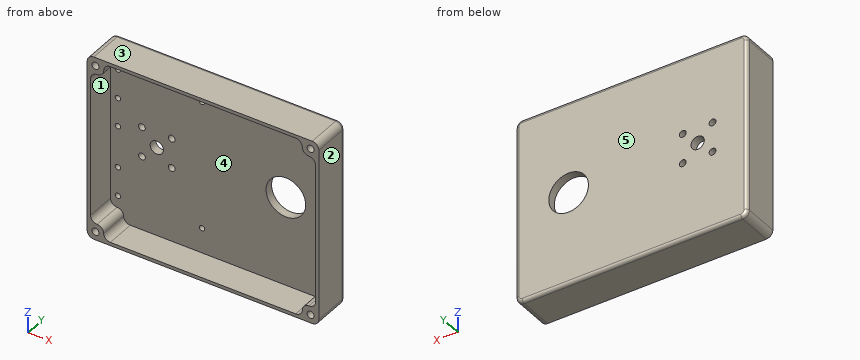
```python
from build123d import *

# Parameters (mm, degrees)
SKETCH2_R           = 3.3734375
BOSS_EXTRUDE1_DEPTH = 28.575
SKETCH2_3_R         = 19.05
SKETCH2_3_R_2       = 3.2639
SKETCH2_3_R_3       = 6.35
BOSS_EXTRUDE2_DEPTH = 7.9375
FILLET1_R           = 3.175
SKETCH3_R           = 2.57937
CUT_EXTRUDE1_DEPTH  = 4.7625


with BuildPart() as part:
    # Sketch2 → Boss-Extrude1 (new body)
    with BuildSketch(Plane(origin=(0, 0, 0), x_dir=(1, 0, 0), z_dir=(0, 1, 0))):
        with BuildLine():
            Line((104.775, -88.9), (-104.775, -88.9))
            ThreePointArc((-104.775, -88.9), (-109.265128061, -87.040128061), (-111.125, -82.55))
            Line((-111.125, -82.55), (-111.125, 82.55))
            ThreePointArc((-111.125, 82.55), (-109.265128061, 87.040128061), (-104.775, 88.9))
            Line((-104.775, 88.9), (104.775, 88.9))
            ThreePointArc((104.775, 88.9), (109.265128061, 87.040128061), (111.125, 82.55))
            Line((111.125, 82.55), (111.125, -82.55))
            ThreePointArc((111.125, -82.55), (109.265128061, -87.040128061), (104.775, -88.9))
        make_face()
        with Locations((-103.1875, -80.9625)):
            Circle(SKETCH2_R, mode=Mode.SUBTRACT)
        with Locations((-103.1875, 80.9625)):
            Circle(SKETCH2_R, mode=Mode.SUBTRACT)
        with Locations((103.1875, 80.9625)):
            Circle(SKETCH2_R, mode=Mode.SUBTRACT)
        with Locations((103.1875, -80.9625)):
            Circle(SKETCH2_R, mode=Mode.SUBTRACT)
        with BuildLine():
            Line((-107.95, -66.675), (-107.95, 66.772716465))
            ThreePointArc((-107.95, 66.772716465), (-106.090128061, 71.262844526), (-101.6, 73.122716465))
            ThreePointArc((-101.6, 73.122716465), (-97.178967915, 74.953967915), (-95.347716465, 79.375))
            ThreePointArc((-95.347716465, 79.375), (-93.487844526, 83.865128061), (-88.997716465, 85.725))
            Line((-88.997716465, 85.725), (88.9, 85.725))
            ThreePointArc((88.9, 85.725), (93.390128061, 83.865128061), (95.25, 79.375))
            ThreePointArc((95.25, 79.375), (97.109871939, 74.884871939), (101.6, 73.025))
            ThreePointArc((101.6, 73.025), (106.090128061, 71.165128061), (107.95, 66.675))
            Line((107.95, 66.675), (107.95, -66.675))
            ThreePointArc((107.95, -66.675), (106.090128061, -71.165128061), (101.6, -73.025))
            ThreePointArc((101.6, -73.025), (97.109871939, -74.884871939), (95.25, -79.375))
            ThreePointArc((95.25, -79.375), (93.390128061, -83.865128061), (88.9, -85.725))
            Line((88.9, -85.725), (-88.9, -85.725))
            ThreePointArc((-88.9, -85.725), (-93.390128061, -83.865128061), (-95.25, -79.375))
            ThreePointArc((-95.25, -79.375), (-97.109871939, -74.884871939), (-101.6, -73.025))
            ThreePointArc((-101.6, -73.025), (-106.090128061, -71.165128061), (-107.95, -66.675))
        make_face(mode=Mode.SUBTRACT)
    extrude(amount=-BOSS_EXTRUDE1_DEPTH)

    # Sketch2<3> → Boss-Extrude2 (add)
    with BuildSketch(Plane(origin=(0, 0, 0), x_dir=(1, 0, 0), z_dir=(0, 1, 0))):
        with BuildLine():
            Line((-104.775, -88.9), (104.775, -88.9))
            ThreePointArc((104.775, -88.9), (109.265128061, -87.040128061), (111.125, -82.55))
            Line((111.125, -82.55), (111.125, 82.55))
            ThreePointArc((111.125, 82.55), (109.265128061, 87.040128061), (104.775, 88.9))
            Line((104.775, 88.9), (-104.775, 88.9))
            ThreePointArc((-104.775, 88.9), (-109.265128061, 87.040128061), (-111.125, 82.55))
            Line((-111.125, 82.55), (-111.125, -82.55))
            ThreePointArc((-111.125, -82.55), (-109.265128061, -87.040128061), (-104.775, -88.9))
        make_face()
        with Locations((60.325, 0)):
            Circle(SKETCH2_3_R, mode=Mode.SUBTRACT)
        with Locations((-77.7875, -14.2875)):
            Circle(SKETCH2_3_R_2, mode=Mode.SUBTRACT)
        with Locations((-49.2125, -14.2875)):
            Circle(SKETCH2_3_R_2, mode=Mode.SUBTRACT)
        with Locations((-63.5, 0)):
            Circle(SKETCH2_3_R_3, mode=Mode.SUBTRACT)
        with Locations((-77.7875, 14.2875)):
            Circle(SKETCH2_3_R_2, mode=Mode.SUBTRACT)
        with Locations((-49.2125, 14.2875)):
            Circle(SKETCH2_3_R_2, mode=Mode.SUBTRACT)
    extrude(amount=BOSS_EXTRUDE2_DEPTH)

    # Fillet1
    fillet1_edges = [part.edges().sort_by_distance(p)[0] for p in [
        (111.125, 7.9375, 0),
        (109.265128061, 7.9375, -87.040128061),
        (0, 7.9375, -88.9),
        (-109.265128061, 7.9375, 87.040128061),
        (0, 7.9375, 88.9),
        (109.265128061, 7.9375, 87.040128061),
        (-109.265128061, 7.9375, -87.040128061),
        (-111.125, 7.9375, 0),
    ]]
    fillet(fillet1_edges, radius=FILLET1_R)

    # Sketch3 → Cut-Extrude1 (cut)
    with BuildSketch(Plane(origin=(0, 0, 0), x_dir=(1, 0, 0), z_dir=(0, 1, 0))):
        with Locations((-20.16125, 61.643858233)):
            Circle(SKETCH3_R)
        with Locations((-20.16125, -61.546141767)):
            Circle(SKETCH3_R)
        with Locations((-100.80625, -61.546141767)):
            Circle(SKETCH3_R)
        with Locations((-100.80625, -33.606141767)):
            Circle(SKETCH3_R)
        with Locations((-100.80625, 33.703858233)):
            Circle(SKETCH3_R)
        with Locations((-100.80625, 61.643858233)):
            Circle(SKETCH3_R)
        with Locations((-100.80625, -6.301141767)):
            Circle(SKETCH3_R)
    extrude(amount=CUT_EXTRUDE1_DEPTH, mode=Mode.SUBTRACT)


solid = part.part
```
Check sheet for the modelled part. Datum: model origin and axes. Units: mm. Face numbers are marked on the shaded views. A direction names the side the tool comes from. Round coordinates to 2 decimals unless told otherwise and drop trailing zeros. One line per item, written item: value. Start each with the question number.
Q1. Thickness scan on line 1 (Z direction, x = -6.5, y = -7.5) (3 decimals); line 2 (X direction, y = -8.5, z = 43) (3 decimals); line 3 (X direction, y = -24, z = -79) (3 decimals). Record the ranges inside material, lowest first.
Q2. Mould release check, pull along X, two halves, no side actions. Record for the marked faces 1, 2 and 3: pulls with the +X half, pulls with the -X half, needs draft (parallel to the pull), parting line crosses it, or undercut.
Q3. Set-up check for the marked faces 4 and 5: record each of +Z, -Z, +X, -X, +Y, -Y from which the full face is reachable in a straight line by a thin tool's end or side.
Q4. Gauge pin test, flat ends, axial feed: pin 1 Ø4 at (x, z) = (-100, 5.5) entering from -Y; pin 2 Ø2.5 at (x, z) = (-101.5, 60.5) entering from -Y. Record the tip position at first contact, or that the pin passes through.
Q5. Cross-section at B-B (z = 0). Give the number of separate pieces and of enclosed holes in the cut face, and give its area (3 significant figures).
Completed:
1. line 1: z = -88.9 to -85.725, 85.725 to 88.9
1. line 2: x = -111.125 to -107.95, 107.95 to 111.125
1. line 3: x = -111.125 to -105.931, -100.444 to -95.359, 95.261 to 100.444, 105.931 to 111.125
2. face 1: undercut
2. face 2: pulls with the +X half
2. face 3: needs draft
3. face 4: -Y
3. face 5: +Z, -Z, +X, -X, +Y
4. pin 1: stops at y = 0
4. pin 2: stops at y = 4.76
5. separate pieces: 3
5. enclosed holes: 0
5. area: 1,540 mm²
